Input: part model. Units: mm. Frame: model coordinates. A direction names the side the tool comes from. Round coordinates to 2 decimals unless told otherwise and drop trailing zeros. Loops run counter-clockwise (first coordinate to the right, second up) from the corner with the lowest first, then second, coordinate; pieces in that order, holes last. Notation, with made-up numbers: (6, 6.25) -> (20, 6.25) arc R12 cw to (20, 25.25) -> close; hole circle Ø8 at (50, 9). An arc over 180 degrees is marked (long way). Answer in a Markdown table with one row per item. Add a question column.
Q1. Reachability of faces 1 (the face through (8, 0, 79)), 2 (the face through (8, 0, 40)), 3 (the face through (169, 0, 0)) from +Z, -Z, +X, -X, +Y, -Y: full face, straight path, thin tool, end or side. Return the list, or none.
Q2. Pin query (flat end, axial travel): pin 1 (3 mm diameter, centred on y = 20.5, z = -49, fed in from +X); pin 2 (9.5 mm diameter, centred on y = 25, z = -65, fed in from -X); pin 3 (1 mm diameter, centred on y = 11.5, z = -20.5, fed in from +X); pin 4 (5 mm diameter, centred on y = 25, z = 65, fed in from +X). Return the tip coordinate at first contact, or that it passes through.
Q3. Mould query, pull axis Y, two halves, no side actions, for faces 4 (the face through (8, 35, 1)), 5 (the face through (118, 0, 52)), 6 (the face through (3.54, -7.1, 3.69)). Classes: pulls with the +Y half, pulls with the -Y half, needs draft (parallel to the pull), parting line crosses it, or undercut.
Q4. Section A-A, the plane y = 25. Output: boundary loops of the cut face in (x, z), and give its area (3 significant figures).
Q5. Section B-B, the plane z = -22. Output: boundary loops of the cut face in (x, y).
Q6. Section D-D, the plane z = 0. Output: boundary loops of the cut face in (x, y), and give its area (3 significant figures).
Q7. Section C-C, the plane x = 129.5. Output: boundary loops of the cut face in (y, z), and give its area (3 significant figures).
Q8. Ray query, L1, parallel to Y at x = 5, z = 0; L2, parallel to Y at x = 11.5, z = 65; L3, parallel to X at y = 30, z = -4.5. Return the intervals inside material, ascending. Write a range as from..to.
```python
from build123d import *

# Parameters (mm, degrees)
SKETCH_1_W                  = 158
SKETCH_1_H                  = 70
EXTRUDE_1_DEPTH             = 16
PATTERN_LINEAR_1_COUNT      = 3
PATTERN_LINEAR_1_PITCH      = 62
PATTERN_LINEAR_2_COUNT      = 2
PATTERN_LINEAR_2_PITCH      = 130
PATTERN_LINEAR_2_COUNT_DIR2 = 2
PATTERN_LINEAR_2_PITCH_DIR2 = 50
SKETCH_9_W                  = 8
SKETCH_9_H                  = 2.5
HOLE_WIZARD_1_D             = 5
HOLE_WIZARD_1_DEPTH         = 8
HOLE_WIZARD_1_TIP           = 1.443375673
CUT_EXTRUDE_1_DEPTH         = 4


with BuildPart() as part:
    # Sketch 1 → Extrude 1 (new body)
    with BuildSketch(Plane(origin=(0, 0, 0), x_dir=(0, 0, -1), z_dir=(1, 0, 0))):
        Rectangle(SKETCH_1_W, SKETCH_1_H)
    extrude(amount=EXTRUDE_1_DEPTH)

    # Sketch 2 → Cut-Revolve 1 (revolve, cut)
    with BuildSketch(Plane.XY.offset(62), mode=Mode.PRIVATE) as cut_revolve_1_sk:
        with BuildLine():
            Line((0, 9.25), (0, 7.5))
            ThreePointArc((0, 7.5), (0.146446609, 7.853553391), (0.5, 8))
            Line((0.5, 8), (6.5, 8))
            Line((6.5, 8), (6.5, 9))
            Line((6.5, 9), (0.25, 9))
            Line((0.25, 9), (0, 9.25))
        make_face()
    cut_revolve_1 = revolve(cut_revolve_1_sk.sketch.rotate(Axis((6.5, 0, 62), (-1, 0, 0)), 270), axis=Axis((6.5, 0, 62), (-1, 0, 0)), mode=Mode.SUBTRACT)

    # Pattern Linear 1: Cut-Revolve 1 ×3
    with Locations(*[(0, 0, -i * PATTERN_LINEAR_1_PITCH) for i in range(1, PATTERN_LINEAR_1_COUNT)]):
        add(cut_revolve_1, mode=Mode.SUBTRACT)

    # Sketch 4 → Revolve 1 (revolve)
    with BuildSketch(Plane.XY, mode=Mode.PRIVATE) as revolve_1_sk:
        Polygon((16, 0), (16, 10), (145.5, 10), (145.5, 31.25), (169, 31.25), (169, 0), align=None)
    revolve(revolve_1_sk.sketch.rotate(Axis((169, 0, 0), (-1, 0, 0)), 270), axis=Axis((169, 0, 0), (-1, 0, 0)))

    # Sketch 5 → Revolve 2 (revolve)
    with BuildSketch(Plane.XY.offset(62), mode=Mode.PRIVATE) as revolve_2_sk:
        Polygon((16, 0), (16, 10), (217.7, 10), (218, 9.7), (218, 0), align=None)
    revolve(revolve_2_sk.sketch.rotate(Axis((218, 0, 62), (-1, 0, 0)), 270), axis=Axis((218, 0, 62), (-1, 0, 0)))

    # Sketch 6 → Revolve 3 (revolve)
    with BuildSketch(Plane.XY.offset(-62), mode=Mode.PRIVATE) as revolve_3_sk:
        Polygon((16, 0), (16, 10), (217.7, 10), (218, 9.7), (218, 0), align=None)
    revolve(revolve_3_sk.sketch.rotate(Axis((218, 0, -62), (-1, 0, 0)), 270), axis=Axis((218, 0, -62), (-1, 0, 0)))

    # Sketch 7 → Cut-Revolve 2 (revolve, cut)
    with BuildSketch(Plane.XY.offset(65), mode=Mode.PRIVATE) as cut_revolve_2_sk:
        Polygon((0, -25), (0, -20), (0.812, -20.812), (15.188, -20.812), (16, -20), (16, -25), align=None)
    cut_revolve_2 = revolve(cut_revolve_2_sk.sketch.rotate(Axis((16, -25, 65), (-1, 0, 0)), 270), axis=Axis((16, -25, 65), (-1, 0, 0)), mode=Mode.SUBTRACT)

    # Pattern Linear 2: Cut-Revolve 2 2 × 2
    with Locations(*[(0, j * PATTERN_LINEAR_2_PITCH_DIR2, -i * PATTERN_LINEAR_2_PITCH) for i in range(PATTERN_LINEAR_2_COUNT) for j in range(PATTERN_LINEAR_2_COUNT_DIR2) if (i, j) != (0, 0)]):
        add(cut_revolve_2, mode=Mode.SUBTRACT)

    # Sketch 9 → Cut-Revolve 3 (revolve, cut)
    with BuildSketch(Plane.XY.offset(40), mode=Mode.PRIVATE) as cut_revolve_3_sk:
        with Locations((4, 1.25)):
            Rectangle(SKETCH_9_W, SKETCH_9_H)
    revolve(cut_revolve_3_sk.sketch.rotate(Axis((8, 0, 40), (-1, 0, 0)), 270), axis=Axis((8, 0, 40), (-1, 0, 0)), mode=Mode.SUBTRACT)

    # Hole Wizard 1
    with Locations(Plane.ZY):
        with Locations((-40, 0)):
            Hole(HOLE_WIZARD_1_D / 2, depth=HOLE_WIZARD_1_DEPTH)
            with Locations((0, 0, -(HOLE_WIZARD_1_DEPTH + HOLE_WIZARD_1_TIP / 2))):  # 120° drill point
                Cone(0, HOLE_WIZARD_1_D / 2, HOLE_WIZARD_1_TIP, mode=Mode.SUBTRACT)

    # Sketch 12 → Cut-Extrude 1 (cut)
    with BuildSketch(Plane(origin=(0, 0, 0), x_dir=(0, 0, -1), z_dir=(1, 0, 0))):
        with BuildLine():
            Line((39.7, -2.5), (40.3, -2.5))
            ThreePointArc((40.3, -2.5), (42.8, 0), (40.3, 2.5))
            Line((40.3, 2.5), (39.7, 2.5))
            ThreePointArc((39.7, 2.5), (37.2, 0), (39.7, -2.5))
        make_face()
    extrude(amount=CUT_EXTRUDE_1_DEPTH, mode=Mode.SUBTRACT)


solid = part.part
```
Answer block:
| question | item | result |
|---|---|---|
| 1 | face 1 | +Z, +X, -X, +Y, -Y |
| 1 | face 2 | -X |
| 1 | face 3 | +X, +Y, -Y |
| 2 | pin 1 | x = 16 |
| 2 | pin 2 | x = 0.25 |
| 2 | pin 3 | x = 169 |
| 2 | pin 4 | through |
| 3 | face 4 | pulls with the +Y half |
| 3 | face 5 | parting line crosses it |
| 3 | face 6 | undercut |
| 4 | outline | (0, -79) -> (16, -79) -> (16, -70) -> (15.19, -69.19) -> (0.81, -69.19) -> (0, -70) -> close; (0, -60) -> (0.81, -60.81) -> (15.19, -60.81) -> (16, -60) -> (16, 60) -> (15.19, 60.81) -> (0.81, 60.81) -> (0, 60) -> close; (0, 70) -> (0.81, 69.19) -> (15.19, 69.19) -> (16, 70) -> (16, 79) -> (0, 79) -> close; (145.5, -18.75) -> (169, -18.75) -> (169, 18.75) -> (145.5, 18.75) -> close |
| 4 | area | 3,140 mm^2 |
| 5 | outline | (0, -35) -> (16, -35) -> (16, 35) -> (0, 35) -> close; (145.5, -22.19) -> (169, -22.19) -> (169, 22.19) -> (145.5, 22.19) -> close |
| 6 | outline | (0, -35) -> (16, -35) -> (16, -10) -> (145.5, -10) -> (145.5, -31.25) -> (169, -31.25) -> (169, 31.25) -> (145.5, 31.25) -> (145.5, 10) -> (16, 10) -> (16, 35) -> (0, 35) -> (0, 9.25) -> (0.25, 9) -> (6.5, 9) -> (6.5, 8) -> (0.5, 8) arc R0.5 ccw to (0, 7.5) -> (0, -7.5) arc R0.5 ccw to (0.5, -8) -> (6.5, -8) -> (6.5, -9) -> (0.25, -9) -> (0, -9.25) -> close |
| 6 | area | 5,170 mm^2 |
| 7 | outline | circle Ø20 at (0, -62); circle Ø20 at (0, 0); circle Ø20 at (0, 62) |
| 7 | area | 942 mm^2 |
| 8 | L1 | -35..-9, -8..8, 9..35 |
| 8 | L2 | -35..-29.19, -20.81..20.81, 29.19..35 |
| 8 | L3 | 0..16, 145.5..169 |
